Print and shaded views of the part. All mm, measured from the part's lowest x, y and z. Round coordinates to 2 decimals unless told otherwise and drop trailing zeros. Write each loop counter-clockwise with the first axis right and the second up, starting at its lowest first coordinate (ties: lowest second). Pieces come first, ordered by that corner, then holes. Notation, with made-up numbers: (33, -20.5) - (91, -20.5) arc R12 cw to (91, -13.5) - close; hole circle Ø7 at (68, -13). An arc over 180 degrees is marked (long way). Put each result on its own line as item: value. Start each with the question number.
Item 1: Cut at B-B (x = 20.5). Give the cut face in (y, z), and give its area (3 significant figures).
Item 2: Cut at A-A (z = 1.6). Give the cut face in (x, y), and give its area (3 significant figures).
Item 3: Pin check, flat tips, straight feed: pin 1 Ø0.9 at (x, z) = (208, 1.5) entering from -Y; pin 2 Ø0.9 at (y, z) = (44, 1.5) entering from +X; pin 3 Ø1.5 at (y, z) = (2, 1.5) entering from -X. Stop position of each tip, or through.
Item 4: Drill centre line: line 1 (Y direction, x = 16.5, z = 0.4). Where is it in solid material? Low to high. Write a range as from..to.
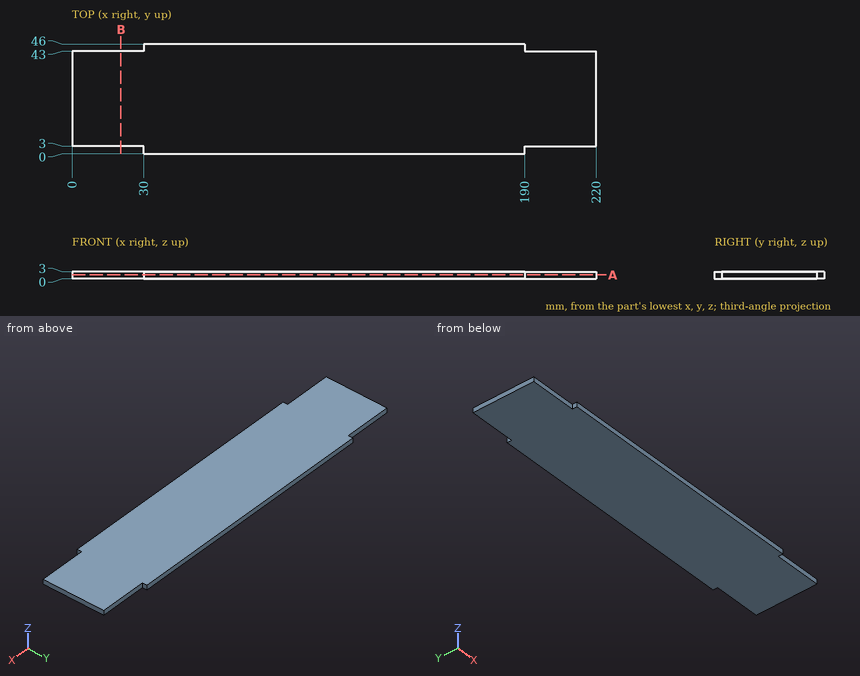
Output values:
1. outline: (3, 0) - (43, 0) - (43, 3) - (3, 3) - close
1. area: 120 mm2
2. outline: (0, 3) - (30, 3) - (30, 0) - (190, 0) - (190, 3) - (220, 3) - (220, 43) - (190, 43) - (190, 46) - (30, 46) - (30, 43) - (0, 43) - close
2. area: 9,760 mm2
3. pin 1: y = 3
3. pin 2: x = 190
3. pin 3: x = 30
4. line 1: 3..43
